Build history of the part. All positions in model axes, mm. A direction names the side the tool comes from. Give positions to 0.01 mm unless a question says otherwise; leave off trailing zeros. Write each loop counter-clockwise with the first axis right and the second up, starting at its lowest first coordinate (ties: lowest second). Pieces come first, ordered by that corner, then holes. Notation, with made-up numbers: (78, -21) -> (131, -21) arc R6 ccw to (131, -14) -> close; hole circle Ø5 at (-7, 35). An arc over 180 degrees is marked (long way). Write item = value, one per line. Start each with the question number.
Q1. Wall check: line 1 (X direction, y = 105, z = -10); line 2 (Y direction, x = -25, z = -4); line 3 (Y direction, x = -25, z = -11). Give the ranges that are in metal, low to high.
Q2. Saw through at C-C, the plane y = 77.5. List the corners of the cut face in (x, z), then the cut area to 3 significant figures.
Q3. Saw through at A-A, the plane x = -28. List the corners of the cut face in (y, z), then the cut area to 3 significant figures.
Q4. Saw through at B-B, the plane z = 36.5. List the corners of the cut face in (x, y), then the cut area to 3 significant figures.
Q5. Mould opens along Z. For faces 1 (the face through (1, 15, -15)), 2 (the face through (-18, 85, 12)), 3 (the face through (1, 30, -13)), 4 (the face through (-0.07, 44.858, 30.363)) say: pulls with the +Z half, pulls with the -Z half, needs draft (parallel to the pull), parting line crosses it, or undercut.
Q6. Saw through at D-D, the plane x = 0. List the corners of the cut face in (y, z).
Q7. Drop flat-ended pins along their axis: P1, Ø20, axis at x = 17.5, z = 14.5, coming from the -Y side; P2, Ø18, axis at x = 14, y = 53.5, coming from the -Z side; P3, Ø11.5, axis at x = -25, y = 15, coming from the +Z side. Give the stop position or say it passes through.
Q8. Tool access for faces 5 (the face through (-5, 60, 18)), 6 (the face through (1, 60, -10)), 7 (the face through (30, 100.2, 36.7)): list every direction of +Z, -Z, +X, -X, +Y, -Y with a clear straight run to the whole face (end or side of a thin tool).
Solid Edge part; units mm, degrees
sketch "Sketch1" plane through (0, 0, 0) normal (0, -1, 0) x (1, 0, 0)
  line L0 (40, 0) -> (40, -15)
  line L1 (40, -15) -> (0, -15)
  line L2 (0, -15) -> (-40, -15)
  line L3 (-40, -15) -> (-40, 0)
  line L4 (-40, 0) -> (0, 0)
  line L5 (0, 0) -> (40, 0)
extrude "Protrusion1" add sketch "Sketch1" against normal blind 120
sketch "Sketch2" plane through (40, 60, -7.5) normal (1, 0, 0) x (0, 1, 0)
  line L0 (-30, -2.5) -> (30, -2.5)
  line L1 (30, -2.5) -> (30, -7.5)
  line L2 (30, -7.5) -> (-30, -7.5)
  line L3 (-30, -7.5) -> (-30, -2.5)
extrude "ExtrudedCutout_1" cut sketch "Sketch2" against normal blind 80
sketch "Sketch3" plane through (0, 0, 0) normal (1, 0, 0) x (0, 1, 0)
  line L0 (95, 0) -> (95, 25.3185)
  line L1 (90, 0) -> (95, 0)
  line L2 (85, 0) -> (90, 0)
  line L3 (85, 0) -> (85, 25.3185)
  arc A0 (85, 25.3185) -> (95, 25.3185) centre (90, 60) cw
extrude "ExtrudedProtrusion_2" add sketch "Sketch3" along normal mid plane 60
sketch "Sketch4" plane through (0, 0, 0) normal (1, 0, 0) x (0, 1, 0)
  circle A0 centre (90, 60) radius 25
extrude "ExtrudedCutout_2" cut sketch "Sketch4" along normal mid plane 60
sketch "Sketch5" plane through (0, 0, 0) normal (1, 0, 0) x (0, 1, 0)
  line L0 (35, 0) -> (54.9959, 61.5877)
  line L1 (55.034, 61.5417) -> (54.9959, 61.5877)
  line L2 (85, 25.3185) -> (84.962, 25.3645)
  line L3 (85, 0) -> (85, 25.3185)
  line L4 (35, 0) -> (85, 0)
  arc A0 (84.962, 25.3645) -> (55.034, 61.5417) centre (90, 60) cw
extrude "ExtrudedProtrusion_3" add sketch "Sketch5" along normal mid plane 10
sketch "Sketch6" plane through (0, 60, 0) normal (0, 0, 1) x (0, 1, 0)
  circle A0 centre (-45, -25) radius 5
extrude "ExtrudedCutout_3" cut sketch "Sketch6" against normal blind 15
sketch "Sketch7" plane through (0, 60, 0) normal (0, 0, 1) x (0, 1, 0)
  circle A0 centre (-45, 25) radius 5
extrude "ExtrudedCutout_4" cut sketch "Sketch7" against normal blind 15
sketch "Sketch8" plane through (0, 60, 0) normal (0, 0, 1) x (0, 1, 0)
  circle A0 centre (45, -25) radius 5
extrude "ExtrudedCutout_5" cut sketch "Sketch8" against normal blind 15
sketch "Sketch9" plane through (0, 60, 0) normal (0, 0, 1) x (0, 1, 0)
  circle A0 centre (45, 25) radius 5
extrude "ExtrudedCutout_6" cut sketch "Sketch9" against normal blind 15
Report:
q1.line_1 = -40 to -30, -20 to 20, 30 to 40
q1.line_2 = 0 to 10, 20 to 100, 110 to 120
q1.line_3 = 0 to 10, 20 to 30, 90 to 100, 110 to 120
q2.outline = (-40, -10) -> (40, -10) -> (40, 0) -> (5, 0) -> (5, 27.27) -> (30, 27.27) -> (30, 38.35) -> (-30, 38.35) -> (-30, 27.27) -> (-5, 27.27) -> (-5, 0) -> (-40, 0) -> close; (-30, 81.65) -> (30, 81.65) -> (30, 92.73) -> (-30, 92.73) -> close
q2.area = 2,400 mm2
q3.outline = (0, -15) -> (11, -15) -> (11, 0) -> (0, 0) -> close; (19, -15) -> (30, -15) -> (30, -10) -> (90, -10) -> (90, -15) -> (101, -15) -> (101, 0) -> (95, 0) -> (95, 25.32) arc R35.04 ccw (long way) to (85, 25.32) -> (85, 0) -> (19, 0) -> close; (109, -15) -> (120, -15) -> (120, 0) -> (109, 0) -> close; hole circle Ø50 at (90, 60)
q3.area = 3,400 mm2
q4.outline = (-30, 64.01) -> (-5, 64.01) -> (-5, 46.85) -> (5, 46.85) -> (5, 64.01) -> (30, 64.01) -> (30, 81.47) -> (-30, 81.47) -> close; (-30, 98.53) -> (30, 98.53) -> (30, 115.99) -> (-30, 115.99) -> close
q4.area = 2,270 mm2
q5.face_1 = pulls with the -Z half
q5.face_2 = undercut
q5.face_3 = needs draft
q5.face_4 = pulls with the +Z half
q6.outline = (0, -15) -> (30, -15) -> (30, -10) -> (90, -10) -> (90, -15) -> (120, -15) -> (120, 0) -> (95, 0) -> (95, 25.32) arc R35.04 ccw (long way) to (55, 61.59) -> (35, 0) -> (0, 0) -> close; hole circle Ø50 at (90, 60)
q7.P1 = 85
q7.P2 = -10
q7.P3 = 0
q8.face_5 = -X, -Y
q8.face_6 = -Z, +X, -X
q8.face_7 = +Z, +X, +Y, -Y
